Design review of the part built by this model. Coordinates are the model's own, in mm. A direction names the side the tool comes from. Coordinates: 2 decimals unless noted, no trailing zeros. Loops run counter-clockwise (first coordinate to the right, second up) from the corner with the lowest first, then second, coordinate; pieces in that order, holes last. Notation, with made-up numbers: (84.25, 77.25) - (94.25, 77.25) arc R7 ccw to (94.25, 81.25) - close; hole circle Ø10 at (84, 1.5). An arc over 180 degrees is marked (long way). Return JSON: item names as keys, results as strings. Group by question number.
from build123d import *

# Parameters (mm, degrees)
BOSS_EXTRUDE1_DEPTH       = 15
SHELL1_T                  = 3
SKETCH3_W                 = 9
SKETCH3_H                 = 11
CUT_EXTRUDE1_DEPTH        = 3
SKETCH4_R                 = 2.5
CUT_EXTRUDE2_DEPTH        = 3
FILLET1_R                 = 2
SKETCH5_R                 = 3
BOSS_EXTRUDE2_DEPTH       = 3.4
SKETCH6_R                 = 1.9
BOSS_EXTRUDE3_DEPTH       = 1.2
SKETCH_PATTERN1_OUTLINE_R = 3
SKETCH_PATTERN1_DEPTH     = 3.4
SKETCH9_W                 = 12
SKETCH9_H                 = 5
BOSS_EXTRUDE4_DEPTH       = 15
SKETCH10_W                = 12
SKETCH10_H                = 5
BOSS_EXTRUDE5_DEPTH       = 5
SKETCH11_W                = 6
SKETCH11_H                = 5
BOSS_EXTRUDE6_DEPTH       = 7
LPATTERN1_COUNT           = 5
LPATTERN1_PITCH           = 10
MIRROR2_COPY_1_SKETCH_W   = 6
MIRROR2_COPY_1_SKETCH_H   = 5
MIRROR2_COPY_1_DEPTH      = 7
MIRROR2_COPY_2_SKETCH_W   = 6
MIRROR2_COPY_2_SKETCH_H   = 5
MIRROR2_COPY_2_DEPTH      = 7
MIRROR2_COPY_3_SKETCH_W   = 6
MIRROR2_COPY_3_SKETCH_H   = 5
MIRROR2_COPY_3_DEPTH      = 7
MIRROR2_COPY_4_SKETCH_W   = 6
MIRROR2_COPY_4_SKETCH_H   = 5
MIRROR2_COPY_4_DEPTH      = 7


# Read off the part's stored shape, not the designer's step: Sketch-Pattern1
with BuildPart() as part:
    # Sketch1 → Boss-Extrude1 (new body)
    with BuildSketch(Plane(origin=(0, 0, 0), x_dir=(1, 0, 0), z_dir=(0, 1, 0))):
        Polygon((0, 0), (88, 0), (88, -41), (71.5, -41), (71.5, -111), (16.5, -111), (16.5, -41), (0, -41), align=None)
    extrude(amount=BOSS_EXTRUDE1_DEPTH)

    # Shell1
    shell1_openings = [part.faces().sort_by_distance(p)[0] for p in [
        (44, 15, 49.150442478),
    ]]
    offset(amount=SHELL1_T, openings=shell1_openings, kind=Kind.INTERSECTION)

    # Sketch3 → Cut-Extrude1 (cut)
    with BuildSketch(Plane(origin=(0, 0, -3), x_dir=(-1, 0, 0), z_dir=(0, 0, -1))):
        with Locations((-62, 9.5)):
            Rectangle(SKETCH3_W, SKETCH3_H)
    extrude(amount=-CUT_EXTRUDE1_DEPTH, mode=Mode.SUBTRACT)

    # Sketch4 → Cut-Extrude2 (cut)
    with BuildSketch(Plane.ZY.offset(3)):
        with Locations((26, 9)):
            Circle(SKETCH4_R)
    extrude(amount=-CUT_EXTRUDE2_DEPTH, mode=Mode.SUBTRACT)

    # Fillet1
    fillet1_edges = [part.edges().sort_by_distance(p)[0] for p in [
        (44, -3, 114),
        (13.5, -3, 79),
        (5.25, -3, 44),
        (-3, -3, 20.5),
        (-3, 6, -3),
        (91, 6, -3),
        (91, 6, 44),
        (74.5, 6, 44),
        (74.5, 6, 114),
        (13.5, 6, 114),
        (13.5, 6, 44),
        (-3, 6, 44),
        (44, -3, -3),
        (91, -3, 20.5),
        (82.75, -3, 44),
        (74.5, -3, 79),
    ]]
    fillet(fillet1_edges, radius=FILLET1_R)

    # Sketch5 → Boss-Extrude2 (add)
    with BuildSketch(Plane(origin=(0, 0, 0), x_dir=(1, 0, 0), z_dir=(0, 1, 0))):
        with Locations(Location((39.5, -80, 0), (0, 0, 90))):
            Circle(SKETCH5_R)
        with Locations(Location((79.5, -20, 0), (0, 0, 90))):
            Circle(SKETCH5_R)
    extrude(amount=BOSS_EXTRUDE2_DEPTH)

    # Sketch6 → Boss-Extrude3 (add)
    with BuildSketch(Plane(origin=(0, 3.4, 0), x_dir=(1, 0, 0), z_dir=(0, 1, 0))):
        with Locations(Location((39.5, -80, 0), (0, 0, 270))):
            Circle(SKETCH6_R)
        with Locations(Location((79.5, -20, 0), (0, 0, 270))):
            Circle(SKETCH6_R)
    extrude(amount=BOSS_EXTRUDE3_DEPTH)

    # Sketch-Pattern1 outline → Sketch-Pattern1 (add)
    with BuildSketch(Plane(origin=(0, 0, 0), x_dir=(1, 0, 0), z_dir=(0, 1, 0))):
        with Locations((63.5, -103)):
            Circle(SKETCH_PATTERN1_OUTLINE_R)
        with Locations((24.5, -103)):
            Circle(SKETCH_PATTERN1_OUTLINE_R)
        with Locations((24.5, -61)):
            Circle(SKETCH_PATTERN1_OUTLINE_R)
        with Locations((47.5, -61)):
            Circle(SKETCH_PATTERN1_OUTLINE_R)
    extrude(amount=SKETCH_PATTERN1_DEPTH)

    # Sketch9 → Boss-Extrude4 (add)
    with BuildSketch(Plane(origin=(0, 0, 0), x_dir=(1, 0, 0), z_dir=(0, 1, 0))):
        with Locations((6, -38.5)):
            Rectangle(SKETCH9_W, SKETCH9_H)
        with Locations((82, -38.5)):
            Rectangle(SKETCH9_W, SKETCH9_H)
    extrude(amount=BOSS_EXTRUDE4_DEPTH)

    # Sketch10 → Boss-Extrude5 (add)
    with BuildSketch(Plane(origin=(0, 0, 36), x_dir=(-1, 0, 0), z_dir=(0, 0, -1))):
        with Locations((-6, 12.5)):
            Rectangle(SKETCH10_W, SKETCH10_H)
    boss_extrude5 = extrude(amount=BOSS_EXTRUDE5_DEPTH)

    # Mirror1: Boss-Extrude5 across plane
    add(boss_extrude5.mirror(Plane.ZY.offset(-44)))

    # Sketch11 → Boss-Extrude6 (add)
    with BuildSketch(Plane.ZY.offset(-71.5)):
        with Locations((108, 12.5)):
            Rectangle(SKETCH11_W, SKETCH11_H)
    boss_extrude6 = extrude(amount=BOSS_EXTRUDE6_DEPTH)

    # LPattern1: Boss-Extrude6 ×5
    with Locations(*[(0, 0, -i * LPATTERN1_PITCH) for i in range(1, LPATTERN1_COUNT)]):
        add(boss_extrude6)

    # Mirror2: Boss-Extrude6 across plane
    add(boss_extrude6.mirror(Plane.ZY.offset(-44)))

    # Mirror2 copy 1 sketch → Mirror2 copy 1 (add)
    with BuildSketch(Plane(origin=(16.5, 0, -10), x_dir=(0, 0, 1), z_dir=(1, 0, 0))):
        with Locations((108, -12.5)):
            Rectangle(MIRROR2_COPY_1_SKETCH_W, MIRROR2_COPY_1_SKETCH_H)
    extrude(amount=MIRROR2_COPY_1_DEPTH)

    # Mirror2 copy 2 sketch → Mirror2 copy 2 (add)
    with BuildSketch(Plane(origin=(16.5, 0, -20), x_dir=(0, 0, 1), z_dir=(1, 0, 0))):
        with Locations((108, -12.5)):
            Rectangle(MIRROR2_COPY_2_SKETCH_W, MIRROR2_COPY_2_SKETCH_H)
    extrude(amount=MIRROR2_COPY_2_DEPTH)

    # Mirror2 copy 3 sketch → Mirror2 copy 3 (add)
    with BuildSketch(Plane(origin=(16.5, 0, -30), x_dir=(0, 0, 1), z_dir=(1, 0, 0))):
        with Locations((108, -12.5)):
            Rectangle(MIRROR2_COPY_3_SKETCH_W, MIRROR2_COPY_3_SKETCH_H)
    extrude(amount=MIRROR2_COPY_3_DEPTH)

    # Mirror2 copy 4 sketch → Mirror2 copy 4 (add)
    with BuildSketch(Plane(origin=(16.5, 0, -40), x_dir=(0, 0, 1), z_dir=(1, 0, 0))):
        with Locations((108, -12.5)):
            Rectangle(MIRROR2_COPY_4_SKETCH_W, MIRROR2_COPY_4_SKETCH_H)
    extrude(amount=MIRROR2_COPY_4_DEPTH)


solid = part.part
Item 1: Add section B-B (z = 26). State the section outline as (x, y) points, then the cut area to 3 significant figures.
Item 2: Add section C-C (x = 47.5). State the section outline as (y, z) points.
Item 3: To check wall thickness, follow line 1 (Z direction, x = 71, y = 12.5); line 2 (X direction, y = 9, z = 94); line 3 (Z direction, x = 45.5, y = 11.25). State the ranges of each line that lie inside material, in increasing order. Write a range as from..to.
Item 4: For faces 5 (the face through (68, 12, 71)), 6 (the face through (68, 10, 98)), 7 (the face through (62, 4, -2)), list the 3-axis set-ups (+Z, -Z, +X, -X, +Y, -Y) from which the entire face can be reached by the end or side of a thin tool; tool diameter is ignored.
Item 5: For P1, Ø6.5, axis at x = 25.5, z = 102, coming from the +Y side; P2, Ø10, axis at x = 7, z = 48.5, coming from the -Y side; P3, Ø4, axis at y = 13, z = 97, coming from the +X side; P4, Ø1.5, axis at y = 13, z = 77, coming from the -X side, all flat-tipped, find the tip position at first contact; note any pin that passes through.
Item 6: Add section A-A (y = 1.5). Give the number of separate pieces and of enclosed holes in the cut face, then the cut area to 3 significant figures.
Item 7: Add section D-D (z = 10). State the section outline as (x, y) points, then the cut area to 3 significant figures.
Item 8: Draft analysis for pull direction Z (two halves, no side actions). For faces 1 (the face through (64.5, 13, 88)), 2 (the face through (24, 3.4, 103)), 3 (the face through (83, 7, 44)), 4 (the face through (80, 4.6, 20)), state which applies: pulls with the +Z half, pulls with the -Z half, needs draft (parallel to the pull), parting line crosses it, or undercut.
Answers below:
{
 "1": {"outline": "(-3, -1) arc R2 ccw to (-1, -3) - (89, -3) arc R2 ccw to (91, -1) - (91, 15) - (88, 15) - (88, 0) - (0, 0) - (0, 6.5) - (-3, 6.5) - close; (-3, 11.5) - (0, 11.5) - (0, 15) - (-3, 15) - close", "area": "355 mm^2"},
 "2": {"outline": "(-3, -1) arc R2 ccw to (-1, -3) - (15, -3) - (15, 0) - (0, 0) - (0, 58) - (3.4, 58) - (3.4, 64) - (0, 64) - (0, 111) - (15, 111) - (15, 114) - (-1, 114) arc R2 ccw to (-3, 112) - close"},
 "3": {"line 1": "z = -3..0, 65..71, 75..81, 85..91, 95..101, 105..114", "line 2": "x = 13.5..16.5, 71.5..74.5", "line 3": "z = -3..0, 111..114"},
 "4": {"face 5": "+Y", "face 6": "none", "face 7": "-Z, +Y"},
 "5": {"P1": "stops at y = 15", "P2": "stops at y = -2.32", "P3": "stops at x = 74.5", "P4": "stops at x = 13.5"},
 "6": {"separate pieces": "7", "enclosed holes": "1", "area": "1,520 mm^2"},
 "7": {"outline": "(-3, -1) arc R2 ccw to (-1, -3) - (89, -3) arc R2 ccw to (91, -1) - (91, 15) - (88, 15) - (88, 0) - (0, 0) - (0, 15) - (-3, 15) - close", "area": "370 mm^2"},
 "8": {"face 1": "needs draft", "face 2": "undercut", "face 3": "pulls with the +Z half", "face 4": "undercut"}
}
